```python
from build123d import *

# Parameters (mm, degrees)
F0_W     = 35.5
F0_H     = 35.5
F1_DEPTH = 60
F2_R     = 8
F3_DEPTH = 50
F5_DEPTH = 30


with BuildPart() as f1:
    # F0 (on Front) → F1 (new body)
    with BuildSketch(Plane.XZ):
        Rectangle(F0_W, F0_H)
    extrude(amount=F1_DEPTH)

    # F2 (on face) → F3 (cut)
    with BuildSketch(Plane(origin=(0, 0, 0), x_dir=(-1, 0, 0), z_dir=(0, 1, 0))):
        Circle(F2_R)
    extrude(amount=-F3_DEPTH, mode=Mode.SUBTRACT)

    # F4 (on face) → F5 (cut)
    with BuildSketch(Plane(origin=(0, 0, 0), x_dir=(-1, 0, 0), z_dir=(0, 1, 0))):
        with BuildLine():
            ThreePointArc((1.5, -7.858117), (0, 8), (-1.5, -7.858117))
            Line((-1.5, -7.858117), (-1.5, -17.75))
            Line((-1.5, -17.75), (1.5, -17.75))
            Line((1.5, -17.75), (1.5, -7.858117))
        make_face()
    extrude(amount=-F5_DEPTH, mode=Mode.SUBTRACT)


solid = f1.part
```
Read the model definition and answer for the solid it produces. Units are mm, in the model's axes. A direction names the side the tool comes from. Give positions to 0.01 mm unless a question says otherwise; leave off trailing zeros. Loops run counter-clockwise (first coordinate to the right, second up) from the corner with the lowest first, then second, coordinate; pieces in that order, holes last.
Item 1: For faces 1 (the flat face through (0, -50, 0)), 2 (the flat face through (1.5, -15, -13)), 3 (the flat face through (-4, -30, -17.75)), determine the directions among +Z, -Z, +X, -X, +Y, -Y from which every point of the face is accessible in a straight line to the end or side of a thin tool.
Item 2: The part is cut by section C-C (y = -37). Write down the section's boundary in (x, z).
Item 3: The part is cut by section B-B (z = 0). Write down the section's boundary in (x, y), and give its area (3 significant figures).
Item 4: The part is cut by section A-A (y = -3.5). Write down the section's boundary in (x, z).
Item 5: Each of these flat-tipped pins is pushed along its axis until it touches: pin 1 Ø5 at (x, z) = (-13, 0) entering from +Y; pin 2 Ø1.5 at (x, z) = (0, -11.5) entering from +Y; pin 3 Ø1.5 at (x, z) = (1, -5.5) entering from +Y. Where does it stop, or does it pass through?
Item 6: The mould has two halves that part along X. Classify faces 4 (the flat face through (0, -30, -13)), 5 (the flat face through (0, -30, 17.75)), 6 (the flat face through (-17.75, -30, 0)), 7 (the flat face through (17.75, -30, 0)): released by +X, released by -X, zero draft, split by the parting line, or undercut.
Item 7: Find the intervals of material crossed by line 1 along X through (y, z) = (-10, 0); line 2 along Z through (x, y) = (0, -26), in increasing order.
Taken from the geometry:
1. face 1: +Y
1. face 2: -Z, +Y
1. face 3: -Z, +X, -X, +Y, -Y
2. outline: (-17.75, -17.75) - (17.75, -17.75) - (17.75, 17.75) - (-17.75, 17.75) - close; hole circle Ø16 at (0, 0)
3. outline: (-17.75, -60) - (17.75, -60) - (17.75, 0) - (8, 0) - (8, -50) - (-8, -50) - (-8, 0) - (-17.75, 0) - close
3. area: 1,330 mm2
4. outline: (-17.75, -17.75) - (-1.5, -17.75) - (-1.5, -7.86) arc R8 cw (long way) to (1.5, -7.86) - (1.5, -17.75) - (17.75, -17.75) - (17.75, 17.75) - (-17.75, 17.75) - close
5. pin 1: stops at y = 0
5. pin 2: stops at y = -30
5. pin 3: stops at y = -50
6. face 4: undercut
6. face 5: zero draft
6. face 6: released by -X
6. face 7: released by +X
7. line 1: x = -17.75 to -8, 8 to 17.75
7. line 2: z = 8 to 17.75
